from build123d import *

# Parameters (mm, degrees)
BOSS_EXTRUDE1_DEPTH = 7
SKETCH3_R           = 5
BOSS_EXTRUDE2_DEPTH = 55
CHAMFER1_SIZE       = 0.75


with BuildPart() as part:
    # Sketch1 → Boss-Extrude1 (new body)
    with BuildSketch(Plane.XY):
        Polygon((9.814954576, 0), (4.907477288, 8.5), (-4.907477288, 8.5), (-9.814954576, 0), (-4.907477288, -8.5), (4.907477288, -8.5), align=None)
    extrude(amount=BOSS_EXTRUDE1_DEPTH)

    # Sketch2 → Cut-Revolve1 (revolve, cut)
    with BuildSketch(Plane(origin=(0, 0, 0), x_dir=(0, 0, -1), z_dir=(1, 0, 0))):
        Polygon((-7, 8.5), (-7, 13.5), (-4.113248654, 13.5), align=None)
    revolve(axis=Axis((0, 0, 7), (0, 0, -1)), mode=Mode.SUBTRACT)

    # Sketch3 → Boss-Extrude2 (add)
    with BuildSketch(Plane(origin=(0, 0, 0), x_dir=(-1, 0, 0), z_dir=(0, 0, -1))):
        with Locations(Location((0, 0, 0), (0, 0, 180))):
            Circle(SKETCH3_R)
    extrude(amount=BOSS_EXTRUDE2_DEPTH)

    # Chamfer1
    chamfer1_edges = [part.edges().sort_by_distance(p)[0] for p in [
        (-5, 0, -55),
    ]]
    chamfer(chamfer1_edges, length=CHAMFER1_SIZE)


solid = part.part
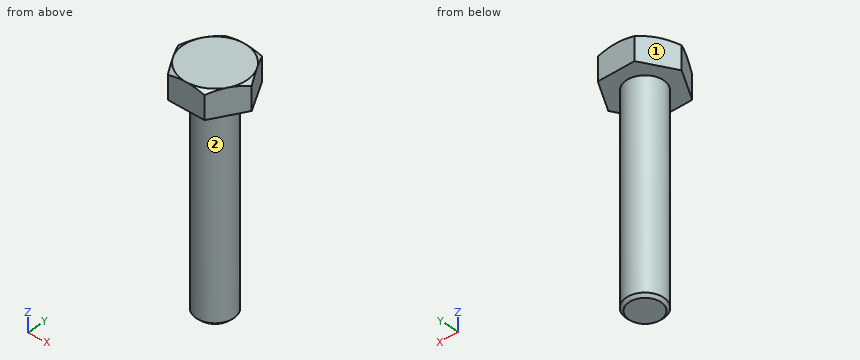
Geometry: final body of the model. Coordinates: model frame, mm. Face numbers are marked on the shaded views. A direction names the side the tool comes from. Coordinates: 2 decimals unless noted, no trailing zeros. Loops run counter-clockwise (first coordinate to the right, second up) from the corner with the lowest first, then second, coordinate; pieces in that order, holes last. Notation, with made-up numbers: M -17,-26.5 L 21,-26.5 A19 ccw 21,-3.5 Z; hole C 58.25,31 d7. An arc over 180 degrees is marked long. One line per item, written item: value. Start each with the question number.
1) Pin query (flat end, axial travel): P1, Ø2, axis at x = 3.5, z = -30, coming from the -Y side; P2, Ø1.5, axis at y = 2, z = -15.5, coming from the -X side; P3, Ø8, axis at x = 0.5, z = -31, coming from the +Y side; P4, Ø1.5, axis at y = -6, z = -35.5, coming from the -X side. Return the tip coordinate at first contact, or that it passes through.
2) Cut plane A-A (z = -3). Return loops of the section in (x, y).
3) Reachability of the marked faces 1 and 2 from +Z, -Z, +X, -X, +Y, -Y: full face, straight path, thin tool, end or side. Return the list, or none.
4) Material intervals for L1, parallel to Z at x = -1.25, y = 6.5; L2, parallel to Y at x = 1, z = -35; L3, parallel to X at y = -2.5, z = 3.5, sorted ascending. Write a range as from..to.
Evaluation:
1. P1: y = -4.33
1. P2: x = -4.84
1. P3: y = 5
1. P4: through
2. outline: C 0,0 d10
3. face 1: +Z, -Z, -X, +Y
3. face 2: -Z
4. L1: 0..7
4. L2: -4.9..4.9
4. L3: -8.37..8.37
